Build history of the part. All positions in model axes, mm. A direction names the side the tool comes from. Give positions to 0.01 mm unless a question says otherwise; leave off trailing zeros. Loops run counter-clockwise (first coordinate to the right, second up) from the corner with the lowest first, then second, coordinate; pieces in that order, holes last. Notation, with made-up numbers: (58.5, -39.75) -> (74.5, -39.75) arc R19 cw to (74.5, -34.75) -> close; hole circle Ø4 at (-28.75, -19). An arc over 180 degrees is marked (long way). Answer as a JSON object with one key per item and string values. Group by question number.
Q1. Two-plate mould, pull along X, no slides. Class faces 1 (the flat face through (-13.5, 0, 1)), 2 (the flat face through (-12, -5, 1)), 3 (the cylindrical face through (10.1, -0.1, 1.5)): pulls with the +X half, pulls with the -X half, needs draft (parallel to the pull), parting line crosses it, or undercut.
Q2. Tool access for faces 4 (the flat face through (-9.26, -3, 1.5)), 5 (the flat face through (-0.2, 0.1, 2)), 6 (the flat face through (4, -2, 1)): list every direction of +Z, -Z, +X, -X, +Y, -Y with a clear straight run to the whole face (end or side of a thin tool).
Q3. Wall check: probe 1 along X at (y, z) = (-3.75, 1.2); probe 2 along X at (y, z) = (-3, 0.95); probe 3 along Z at (x, y) = (-11.5, -1.75). Give the ranges that are in metal, low to high. Write a range as from..to.
Q4. Band-saw the part on A-A, the plane y = -2. Count the separate pieces of the cut face and the enclosed holes in it, plus the area to 3 significant figures.
Q5. Band-saw the part on B-B, the plane x = -10.16. Write the cut outline in (y, z), plus the area to 3 significant figures.
from build123d import *

# Parameters (mm, degrees)
F1_DEPTH = 2
F3_DEPTH = 1


with BuildPart() as f1:
    # F0 (on Top) → F1 (new body)
    with BuildSketch(Plane.XY):
        with BuildLine():
            Line((13.5, 5), (-13.5, 5))
            Line((-13.5, 5), (-13.5, -5))
            Line((-13.5, -5), (-11.06, -5))
            Line((-11.06, -5), (-11.06, -1))
            ThreePointArc((-11.06, -1), (-10.16, -0.1), (-9.26, -1))
            Line((-9.26, -1), (-9.26, -5))
            Line((-9.26, -5), (-5.98, -5))
            Line((-5.98, -5), (-5.98, -1))
            ThreePointArc((-5.98, -1), (-5.08, -0.1), (-4.18, -1))
            Line((-4.18, -1), (-4.18, -5))
            Line((-4.18, -5), (-0.9, -5))
            Line((-0.9, -5), (-0.9, -1))
            ThreePointArc((-0.9, -1), (0, -0.1), (0.9, -1))
            Line((0.9, -1), (0.9, -5))
            Line((0.9, -5), (4.18, -5))
            Line((4.18, -5), (4.18, -1))
            ThreePointArc((4.18, -1), (5.08, -0.1), (5.98, -1))
            Line((5.98, -1), (5.98, -5))
            Line((5.98, -5), (9.26, -5))
            Line((9.26, -5), (9.26, -1))
            ThreePointArc((9.26, -1), (10.16, -0.1), (11.06, -1))
            Line((11.06, -1), (11.06, -5))
            Line((11.06, -5), (13.5, -5))
            Line((13.5, -5), (13.5, 5))
        make_face()
    extrude(amount=F1_DEPTH)

    # F2 (on face) → F3 (cut)
    with BuildSketch(Plane(origin=(0, 0, 0), x_dir=(1, 0, 0), z_dir=(0, 0, -1))):
        with BuildLine():
            Line((-11.56, 6.848881), (-11.56, 5))
            Line((-11.56, 5), (-11.56, 1))
            ThreePointArc((-11.56, 1), (-10.16, -0.4), (-8.76, 1))
            Line((-8.76, 1), (-8.76, 5))
            Line((-8.76, 5), (-6.48, 5))
            Line((-6.48, 5), (-6.48, 1))
            ThreePointArc((-6.48, 1), (-5.08, -0.4), (-3.68, 1))
            Line((-3.68, 1), (-3.68, 5))
            Line((-3.68, 5), (-1.4, 5))
            Line((-1.4, 5), (-1.4, 1))
            ThreePointArc((-1.4, 1), (0, -0.4), (1.4, 1))
            Line((1.4, 1), (1.4, 5))
            Line((1.4, 5), (3.68, 5))
            Line((3.68, 5), (3.68, 1))
            ThreePointArc((3.68, 1), (5.08, -0.4), (6.48, 1))
            Line((6.48, 1), (6.48, 5))
            Line((6.48, 5), (8.76, 5))
            Line((8.76, 5), (8.76, 1))
            ThreePointArc((8.76, 1), (10.16, -0.4), (11.56, 1))
            Line((11.56, 1), (11.56, 5))
            Line((11.56, 5), (11.56, 6.848881))
            Line((11.56, 6.848881), (-11.56, 6.848881))
        make_face()
    extrude(amount=-F3_DEPTH, mode=Mode.SUBTRACT)


solid = f1.part
Worked answers:
{
 "1": {"face 1": "pulls with the -X half", "face 2": "needs draft", "face 3": "undercut"},
 "2": {"face 4": "+Z, -Z, -Y", "face 5": "+Z, +X, -X, +Y, -Y", "face 6": "-Z, -Y"},
 "3": {"probe 1": "-13.5..-11.06, -9.26..-5.98, -4.18..-0.9, 0.9..4.18, 5.98..9.26, 11.06..13.5", "probe 2": "-13.5..-11.56, -8.76..-6.48, -3.68..-1.4, 1.4..3.68, 6.48..8.76, 11.56..13.5", "probe 3": "1..2"},
 "4": {"separate pieces": "6", "enclosed holes": "0", "area": "31.0 mm2"},
 "5": {"outline": "(-0.1, 1) -> (0.4, 1) -> (0.4, 0) -> (5, 0) -> (5, 2) -> (-0.1, 2) -> close", "area": "9.70 mm2"}
}
